For this review, take the finished solid that the model builds, in its own axes (mm). A direction names the side the tool comes from. Round coordinates to 2 decimals unless told otherwise and drop trailing zeros. Write each loop counter-clockwise with the first axis right and the second up, starting at its lowest first coordinate (ties: lowest second). Pieces come first, ordered by that corner, then holes. Notation, with made-up numbers: (-8, -26) - (29, -26) arc R24 cw to (29, -9) - close; hole circle Ø10 at (-10.75, -36.5). An arc over 180 degrees is marked (long way). One line per item, written item: value. Start each with the question number.
Q1. Tool access review of faces 1 (the face through (453, 10, 580)), 2 (the face through (328, -740, 442)), 3 (the face through (35, -740, 805)): name each direction out of +Z, -Z, +X, -X, +Y, -Y from which nothing blocks a thin tool from reaching the whole face with its end or side.
Q2. Add section B-B on x = 242. Write out the cut boundary in (y, z), and give its area (3 significant figures).
Q3. Add section A-A on y = -230. Write out the cut boundary in (x, z).
Q4. Clearance check with flat-ended pins moving along their axes: pin 1 Ø10 at (y, z) = (296, 433.5) entering from -X; pin 2 Ø1.5 at (x, y) = (259, 472.5) entering from +Z; pin 3 Ø3 at (y, z) = (-0.5, 240) entering from +X. State where each tip first meets the part, or that it passes through.
Q5. For probe 1 along Z at (x, y) = (31.5, 641); probe 2 along Z at (x, y) = (455.5, -362); probe 3 along Y at (x, z) = (483, 126), list the stretches that pass through material, from the lowest coordinate up.
Q6. Add section D-D on z = 846. Write out the cut boundary in (x, y), and give its area (3 significant figures).
Q7. Add section C-C on z = 472.5. Write out the cut boundary in (x, y), and give its area (3 significant figures).
Q8. Mouldability with a two-part tool opening along X and no side actions: class faces 4 (the face through (619.44, -745.07, 392.8)), 5 (the face through (80, 0, 39)), 6 (the face through (625, 35, 39)), 7 (the face through (650, 10, 141)) as +X half, -X half, draft (parallel to the pull), parting line (faces both ways), or undercut.
Autodesk Inventor part; units mm, degrees
ref_plane "YZ Plane" through (0, 0, 0) normal (1, 0, 0) x (0, 1, 0)
ref_plane "XZ Plane" through (0, 0, 0) normal (0, 1, 0) x (-1, 0, 0)
ref_plane "XY Plane" through (0, 0, 0) normal (0, 0, 1) x (1, 0, 0)
sketch "Sketch1" plane through (0, 0, 0) normal (0, 1, 0) x (-1, 0, 0)
  line L0 (0, 0) -> (0, 1550)
  line L1 (0, 1550) -> (-100, 1550)
  line L2 (-100, 1550) -> (-100, 590)
  line L3 (-100, 590) -> (-580, 590)
  line L4 (-580, 590) -> (-660, 190)
  line L5 (-660, 190) -> (-660, 0)
  line L6 (-660, 0) -> (0, 0)
  dimension "d0" = 1550
  dimension "d1" = 100
  dimension "d2" = 660
  dimension "d3" = 190
  dimension "d4" = 480
  dimension "d5" = 590
extrude "Extrusion1" add sketch "Sketch1" along normal mid plane 1500
sketch "Sketch2" plane through (660, 750, 0) normal (0, 0, -1) x (-1, 0, 0)
  line L0 (0, -1500) -> (0, 0)
  line L1 (660, -1500) -> (0, -1500)
  line L2 (660, -1500) -> (660, 0)
  line L3 (0, 0) -> (660, 0)
  line L4 (0, -1500) -> (0, 0)
  line L5 (0, -1500) -> (70, -1500)
  line L6 (70, -1500) -> (70, -1430)
  line L7 (70, -1430) -> (0, -1430)
  line L8 (0, -1430) -> (0, -1500)
  line L9 (0, -785) -> (70, -785)
  line L10 (70, -785) -> (70, -715)
  line L11 (70, -715) -> (0, -715)
  line L12 (0, -715) -> (0, -785)
  line L13 (0, -70) -> (70, -70)
  line L14 (70, -70) -> (70, 0)
  line L15 (70, 0) -> (0, 0)
  line L16 (0, 0) -> (0, -70)
  line L17 (510, -1500) -> (580, -1500)
  line L18 (580, -1500) -> (580, -1430)
  line L19 (580, -1430) -> (510, -1430)
  line L20 (510, -1430) -> (510, -1500)
  line L21 (510, -785) -> (580, -785)
  line L22 (580, -785) -> (580, -715)
  line L23 (580, -715) -> (510, -715)
  line L24 (510, -715) -> (510, -785)
  line L25 (510, -70) -> (580, -70)
  line L26 (580, -70) -> (580, 0)
  line L27 (580, 0) -> (510, 0)
  line L28 (510, 0) -> (510, -70)
  point P0 (660, -750)
  point P1 (70, 0)
  point P2 (0, -715)
  point P3 (0, -1430)
  point P4 (70, -1500)
  dimension "d8" = 70
  dimension "d9" = 70
  dimension "d20" = 715
  dimension "d23" = 510
extrude "Extrusion2" cut sketch "Sketch2" against normal blind 80 contours L0 L9 L10 L11 L13 L14 L3 L28 L25 L26 L2 L1 L18 L19 L20 L6 L7
sketch "Sketch3" plane through (0, -750, 1550) normal (-1, 0, 0) x (0, 0, 1)
  line L0 (0, 1500) -> (0, 0)
  line L1 (-1470, 1500) -> (0, 1500)
  line L2 (0, 0) -> (-1470, 0)
  line L3 (-1470, 1500) -> (-1470, 0)
  line L4 (-10, 1490) -> (-1460, 1490)
  line L5 (-1460, 1490) -> (-1460, 10)
  line L6 (-1460, 10) -> (-10, 10)
  line L7 (-10, 10) -> (-10, 1490)
  point P0 (-1550, 750)
  dimension "d28" = 10
  dimension "d30" = 10
  dimension "d31" = 10
  dimension "d32" = 10
extrude "Extrusion3" cut sketch "Sketch3" against normal blind 70 contours L7 L6 L5 L4
sketch "Sketch4" plane through (0, -750, 0) normal (0, -1, 0) x (1, 0, 0)
  line L0 (120, 440) -> (480, 440)
  line L1 (500, 420) -> (500, 210)
  line L2 (480, 190) -> (120, 190)
  line L3 (100, 210) -> (100, 420)
  line L4 (0, 1550) -> (0, 80)
  line L5 (150, 80) -> (590, 80)
  arc A0 (120, 440) -> (100, 420) centre (120, 420) ccw
  arc A1 (100, 210) -> (120, 190) centre (120, 210) ccw
  arc A2 (480, 190) -> (500, 210) centre (480, 210) ccw
  arc A3 (500, 420) -> (480, 440) centre (480, 420) ccw
  point P0 (0, 0)
  point P1 (100, 440)
  point P2 (500, 190)
  point P3 (500, 440)
  dimension "d35" = 400
  dimension "d36" = 250
  dimension "d37" = 100
  dimension "d38" = 110
  dimension "d39" = 20
extrude "Extrusion4" cut sketch "Sketch4" against normal through all
sketch "Sketch5" plane through (660, -750, 190) normal (1, 0, 0) x (0, 0, -1)
  line L0 (-1350, 10) -> (0, 10)
  line L1 (0, 10) -> (0, 1490)
  line L2 (0, 1490) -> (-1350, 1490)
  line L3 (-1350, 1490) -> (-1350, 10)
  line L4 (-1360, 1500) -> (-400, 1500)
  line L5 (-400, 0) -> (-1360, 0)
  line L6 (-1360, 0) -> (-1360, 1500)
  line L7 (0, 0) -> (0, 1500)
  point P0 (190, 750)
  point P1 (0, 750)
  point P2 (0, 750)
  dimension "d42" = 10
  dimension "d43" = 10
  dimension "d44" = 10
extrude "Extrusion5" cut sketch "Sketch5" against normal blind 580
sketch "Sketch6" plane through (120, -750, 190) normal (0, 0, 1) x (1, 0, 0)
  line L0 (-40, 1490) -> (530, 1490)
  line L1 (530, 1490) -> (530, 10)
  line L2 (530, 10) -> (-40, 10)
  line L3 (-40, 10) -> (-40, 1490)
  line L4 (540, 10) -> (540, 1490)
  line L5 (-20, 0) -> (-20, 1500)
  line L6 (-50, 10) -> (-50, 1490)
  point P0 (-120, 750)
  point P1 (245, 1490)
  point P2 (460, 1490)
  point P3 (245, 10)
  point P4 (460, 10)
  dimension "d47" = 10
  dimension "d50" = 10
extrude "Extrusion6" cut sketch "Sketch6" against normal blind 100
sketch "Sketch8" plane through (100, 740, 590) normal (0, -1, 0) x (1, 0, 0)
  line L0 (230, -10) -> (480, -10)
  line L1 (480, -10) -> (480, -20)
  line L2 (480, -20) -> (230, -20)
  line L3 (230, -20) -> (230, -10)
  line L4 (240, -20) -> (250, -20)
  line L5 (250, -20) -> (250, -70)
  line L6 (250, -70) -> (240, -70)
  line L7 (240, -70) -> (240, -20)
  line L8 (460, -20) -> (470, -20)
  line L9 (470, -20) -> (470, -70)
  line L10 (470, -70) -> (460, -70)
  line L11 (460, -70) -> (460, -20)
  line L12 (0, 0) -> (480, 0)
  point P0 (-100, -590)
  point P1 (480, -15)
  point P2 (470, -20)
  point P3 (250, -20)
  dimension "d51" = 250
  dimension "d52" = 10
  dimension "d53" = 10
  dimension "d54" = 10
  dimension "d55" = 10
  dimension "d56" = 10
  dimension "d57" = 50
  dimension "d58" = 10
extrude "Extrusion7" add sketch "Sketch8" along normal blind 1480
equation "\"d53\" = d52"
equation "\"d54\" = d52"
properties part number "Стол приёма ГПХ"
Result set:
1. face 1: +Z, +X
1. face 2: none
1. face 3: -X
2. outline: (-750, 80) - (750, 80) - (750, 190) - (740, 190) - (740, 90) - (-740, 90) - (-740, 190) - (-750, 190) - close; (-750, 440) - (-740, 440) - (-740, 590) - (-750, 590) - close; (740, 440) - (750, 440) - (750, 590) - (740, 590) - close
2. area: 20,000 mm^2
3. outline: (0, 80) - (660, 80) - (660, 190) - (650, 190) - (650, 90) - (80, 90) - (80, 1540) - (100, 1540) - (100, 1550) - (0, 1550) - (0, 1540) - (70, 1540) - (70, 90) - (0, 90) - close; (330, 570) - (340, 570) - (340, 520) - (350, 520) - (350, 570) - (560, 570) - (560, 520) - (570, 520) - (570, 570) - (580, 570) - (580, 580) - (330, 580) - close
4. pin 1: stops at x = 70
4. pin 2: stops at z = 90
4. pin 3: stops at x = 80
5. probe 1: z = 80 to 90, 1540 to 1550
5. probe 2: z = 80 to 90, 570 to 580
5. probe 3: y = -750 to -740, 740 to 750
6. outline: (0, -750) - (100, -750) - (100, -740) - (80, -740) - (80, 740) - (100, 740) - (100, 750) - (0, 750) - (0, 740) - (70, 740) - (70, -740) - (0, -740) - close
6. area: 16,800 mm^2
7. outline: (0, -750) - (603.5, -750) - (603.5, -740) - (80, -740) - (80, 740) - (603.5, 740) - (603.5, 750) - (0, 750) - (0, 740) - (70, 740) - (70, -740) - (0, -740) - close
7. area: 26,900 mm^2
8. face 4: +X half
8. face 5: -X half
8. face 6: draft
8. face 7: undercut
